from build123d import *

# Parameters (mm, degrees)
SKETCH2_W                      = 100
SKETCH2_H                      = 100
BOSS_EXTRUDE1_DEPTH            = 2.5
M2_CLEARANCE_HOLE1_D           = 2.4
M2_CLEARANCE_HOLE1_CSINK_D     = 2.45
M2_CLEARANCE_HOLE1_CSINK_ANGLE = 90
LPATTERN1_COUNT                = 3
LPATTERN1_PITCH                = 35
MIRROR1_COPY_1_D               = 2.4
MIRROR1_COPY_1_CSINK_D         = 2.45
MIRROR1_COPY_1_CSINK_ANGLE     = 90
MIRROR1_COPY_2_D               = 2.4
MIRROR1_COPY_2_CSINK_D         = 2.45
MIRROR1_COPY_2_CSINK_ANGLE     = 90
CUT_EXTRUDE1_DEPTH             = 2.5


with BuildPart() as part:
    # Sketch2 → Boss-Extrude1 (new body)
    with BuildSketch(Plane(origin=(0, 0, 0), x_dir=(1, 0, 0), z_dir=(0, 1, 0))):
        Rectangle(SKETCH2_W, SKETCH2_H)
    extrude(amount=BOSS_EXTRUDE1_DEPTH)

    # M2 Clearance Hole1 (through all)
    with Locations(Plane(origin=(0, 2.5, 0), x_dir=(1, 0, 0), z_dir=(0, 1, 0))):
        with Locations((-45.75, 35)):
            m2_clearance_hole1 = CounterSinkHole(M2_CLEARANCE_HOLE1_D / 2, M2_CLEARANCE_HOLE1_CSINK_D / 2, counter_sink_angle=M2_CLEARANCE_HOLE1_CSINK_ANGLE)

    # LPattern1: M2 Clearance Hole1 ×3
    with Locations(*[(0, 0, i * LPATTERN1_PITCH) for i in range(1, LPATTERN1_COUNT)]):
        add(m2_clearance_hole1, mode=Mode.SUBTRACT)

    # Mirror1: M2 Clearance Hole1 across plane
    add(m2_clearance_hole1.mirror(Plane(origin=(0, 0, 0), x_dir=(0, 0, 1), z_dir=(1, 0, 0))), mode=Mode.SUBTRACT)

    # Mirror1 copy 1 (through all)
    with Locations(Plane(origin=(0, 2.5, 35), x_dir=(-1, 0, 0), z_dir=(0, 1, 0))):
        with Locations((-45.75, -35)):
            CounterSinkHole(MIRROR1_COPY_1_D / 2, MIRROR1_COPY_1_CSINK_D / 2, counter_sink_angle=MIRROR1_COPY_1_CSINK_ANGLE)

    # Mirror1 copy 2 (through all)
    with Locations(Plane(origin=(0, 2.5, 70), x_dir=(-1, 0, 0), z_dir=(0, 1, 0))):
        with Locations((-45.75, -35)):
            CounterSinkHole(MIRROR1_COPY_2_D / 2, MIRROR1_COPY_2_CSINK_D / 2, counter_sink_angle=MIRROR1_COPY_2_CSINK_ANGLE)

    # Sketch5 → Cut-Extrude1 (cut)
    with BuildSketch(Plane(origin=(0, 2.5, 0), x_dir=(1, 0, 0), z_dir=(0, 1, 0))):
        with BuildLine():
            Line((1.377777778, 8.309393123), (28.989112389, 34.550266095))
            ThreePointArc((28.989112389, 34.550266095), (29.468680542, 36.741799228), (27.611334612, 38))
            Line((27.611334612, 38), (-27.611334612, 38))
            ThreePointArc((-27.611334612, 38), (-29.468680542, 36.741799228), (-28.989112389, 34.550266095))
            Line((-28.989112389, 34.550266095), (-1.377777778, 8.309393123))
            ThreePointArc((-1.377777778, 8.309393123), (0, 7.759127028), (1.377777778, 8.309393123))
        make_face()
        with BuildLine():
            Line((27.611334612, -38), (-27.611334612, -38))
            ThreePointArc((-27.611334612, -38), (-29.468680542, -36.741799228), (-28.989112389, -34.550266095))
            Line((-28.989112389, -34.550266095), (-1.377777778, -8.309393123))
            ThreePointArc((-1.377777778, -8.309393123), (0, -7.759127028), (1.377777778, -8.309393123))
            Line((1.377777778, -8.309393123), (28.989112389, -34.550266095))
            ThreePointArc((28.989112389, -34.550266095), (29.468680542, -36.741799228), (27.611334612, -38))
        make_face()
        with BuildLine():
            Line((-36, 28.932797546), (-36, -28.932797546))
            ThreePointArc((-36, -28.932797546), (-34.686074143, -30.811441278), (-32.47069773, -30.221686435))
            Line((-32.47069773, -30.221686435), (-8.086269602, -1.288888889))
            ThreePointArc((-8.086269602, -1.288888889), (-7.615571872, 0), (-8.086269602, 1.288888889))
            Line((-8.086269602, 1.288888889), (-32.47069773, 30.221686435))
            ThreePointArc((-32.47069773, 30.221686435), (-34.686074143, 30.811441278), (-36, 28.932797546))
        make_face()
        with BuildLine():
            Line((32.47069773, -30.221686435), (8.086269602, -1.288888889))
            ThreePointArc((8.086269602, -1.288888889), (7.615571872, 0), (8.086269602, 1.288888889))
            Line((8.086269602, 1.288888889), (32.47069773, 30.221686435))
            ThreePointArc((32.47069773, 30.221686435), (34.686074143, 30.811441278), (36, 28.932797546))
            Line((36, 28.932797546), (36, -28.932797546))
            ThreePointArc((36, -28.932797546), (34.686074143, -30.811441278), (32.47069773, -30.221686435))
        make_face()
    extrude(amount=-CUT_EXTRUDE1_DEPTH, mode=Mode.SUBTRACT)


solid = part.part
Could you check a few things on this model? Use its own coordinates, in mm. A direction names the side the tool comes from. Coordinates: 2 decimals unless noted, no trailing zeros. Write each loop counter-clockwise with the first axis right and the second up, starting at its lowest first coordinate (ties: lowest second). Pieces come first, ordered by that corner, then holes. Notation, with made-up numbers: (52.25, 65.5) - (63.25, 65.5) arc R21 cw to (63.25, 87.5) - close; hole circle Ø6 at (57.25, 27.5). An arc over 180 degrees is marked (long way). Write item = value, one per line.
1) Will this pin go through, and if not, where does the flat tip stop? pin 1 Ø6 at (x, z) = (6, 36.5) entering from -Y.
Result set:
pin_1 = 0
2) Suppose I cut it at B-B on x = 45.75. Please give me the cut outline in (y, z) (3 decimals), plus the area to 3 significant figures.
Result set:
outline = (0, -50) - (2.5, -50) - (2.5, -36.225) - (2.475, -36.2) - (0, -36.2) - close; (0, -33.8) - (2.475, -33.8) - (2.5, -33.775) - (2.5, -1.225) - (2.475, -1.2) - (0, -1.2) - close; (0, 1.2) - (2.475, 1.2) - (2.5, 1.225) - (2.5, 33.775) - (2.475, 33.8) - (0, 33.8) - close; (0, 36.2) - (2.475, 36.2) - (2.5, 36.225) - (2.5, 50) - (0, 50) - close
area = 232 mm2
3) We'd pull the mould along Z, two halves only. Please class faces 1 (the flat face through (-50, 1, 1)), 2 (the flat face through (14.99, 1.268, 21.246)): +Z half, -Z half, draft (parallel to the pull), parting line (faces both ways), or undercut.
Result set:
face_1 = draft
face_2 = undercut
4) Suppose I cut it at D-D on z = 12.5. Please give me the cut outline in (x, y).
Result set:
outline = (-50, 0) - (-36, 0) - (-36, 2.5) - (-50, 2.5) - close; (-17.53, 0) - (-5.79, 0) - (-5.79, 2.5) - (-17.53, 2.5) - close; (5.79, 0) - (17.53, 0) - (17.53, 2.5) - (5.79, 2.5) - close; (36, 0) - (50, 0) - (50, 2.5) - (36, 2.5) - close
5) Please list where these lines run through material, in increasing order: line 1 (Z direction, x = -45.75, y = 1.25); line 2 (Z direction, x = 21, y = 1.25); line 3 (X direction, y = 1, z = 35). Write a range as [from, to].
Result set:
line_1 = [-50, -36.2], [-33.8, -1.2], [1.2, 33.8], [36.2, 50]
line_2 = [-50, -38], [-26.96, -16.61], [16.61, 26.96], [38, 50]
line_3 = [-50, -46.95], [-44.55, -29.34], [29.34, 44.55], [46.95, 50]
6) Suppose I cut it at C-C on y = 0.65. State how many separate pieces and enclosed holes the cut face has, plus the area to 3 significant figures.
Result set:
separate_pieces = 1
enclosed_holes = 10
area = 6,000 mm2
7) Suppose I cut it at A-A on z = 0. Please give me the cut outline in (x, y) (3 decimals), plus the area to 3 significant figures.
Result set:
outline = (-50, 0) - (-46.95, 0) - (-46.95, 2.475) - (-46.975, 2.5) - (-50, 2.5) - close; (-44.55, 0) - (-36, 0) - (-36, 2.5) - (-44.525, 2.5) - (-44.55, 2.475) - close; (-7.616, 0) - (7.616, 0) - (7.616, 2.5) - (-7.616, 2.5) - close; (36, 0) - (44.55, 0) - (44.55, 2.475) - (44.525, 2.5) - (36, 2.5) - close; (46.95, 0) - (50, 0) - (50, 2.5) - (46.975, 2.5) - (46.95, 2.475) - close
area = 96.1 mm2
8) For faces 3 (the flat face through (-1, 0, -1)), 4 (the flat face through (-20.45, 1.27, 15.96)), which set-ups out of +Z, -Z, +X, -X, +Y, -Y let a thin tool reach every point of the face, with its end or its side?
Result set:
face_3 = +Z, -Z, +X, -X, -Y
face_4 = +Y, -Y
